Part model, mm, in its own coordinate system. A direction names the side the tool comes from. Coordinates: 2 decimals unless noted, no trailing zeros. Loops run counter-clockwise (first coordinate to the right, second up) from the corner with the lowest first, then second, coordinate; pieces in that order, holes last. Notation, with made-up numbers: (2, -37.5) -> (37, -37.5) arc R9 cw to (37, -27.5) -> close; hole circle Ø1 at (24, 54). An arc over 180 degrees is marked (long way). Use one line per item in the form item = value. Start each with the question number.
(1) Band-saw the part on C-C on y = 26. Give the cut face in (x, z).
(2) 3-axis set-ups, long thin cutter, end or side, ignore diameter. For faces 5 (the flat face through (42.92, 19.18, -0.03)), 6 (the flat face through (43, 32, 0)): which of +Z, -Z, +X, -X, +Y, -Y reach the whole face in a straight line?
(3) Band-saw the part on D-D on x = 14. Give the cut face in (y, z), then the cut area to 3 significant figures.
(4) Mould opens along X. For faces 1 (the cylindrical face through (48.7, 21.833, -0.028)), 2 (the flat face through (24, 18, 2)), 3 (the cylindrical face through (18.821, 14.546, 0.028)), 4 (the flat face through (52.17, 24.97, -0.03)) say: +X half, -X half, draft (parallel to the pull), parting line (faces both ways), or undercut.
(5) Pin check, flat tip, straight feed: P1, Ø3, axis at x = 0, y = 0, coming from the +Z side. Stop position of the tip, or through.
(6) Drill centre lines: L1, parallel to X at y = 27, z = -1.45; L2, parallel to Y at x = 3, z = 0.3; L3, parallel to X at y = 20, z = -0.65. Where is each one in solid material? Low to high. Write a range as [from, to].
(7) Band-saw the part on B-B on x = 0. Give the cut face in (y, z).
(8) Band-saw the part on A-A on z = -1.1. Give the cut face in (x, y), then the cut area to 3 significant figures.
```python
from build123d import *

# Parameters (mm, degrees)
BOSS_EXTRUDE1_DEPTH      = 2
BOSS_EXTRUDE1_DEPTH_BACK = 2
SKETCH2_R                = 1.55
FILLET1_R                = 20
BOSS_EXTRUDE3_START      = -4
BOSS_EXTRUDE3_DEPTH      = 4
FILLET3_R                = 6


with BuildPart() as part:
    # Sketch2 → Boss-Extrude1 (new, two sides: drawn at the far end of the back side and taken through both)
    with BuildSketch(Plane.XY.offset(-BOSS_EXTRUDE1_DEPTH_BACK)):
        with BuildLine():
            Line((1.575752274, -4.745208612), (38.598254294, 14.069940073))
            Line((38.598254294, 14.069940073), (44.683748534, 21.26396825))
            ThreePointArc((44.683748534, 21.26396825), (46.605489471, 28.139740122), (40.590896347, 31.986036602))
            Line((40.590896347, 31.986036602), (3, 31))
            ThreePointArc((3, 31), (-1.722747684, 24.35815521), (6.101607472, 22.078261726))
            Line((6.101607472, 22.078261726), (26.170960727, 22.604695486))
            Line((26.170960727, 22.604695486), (19.115779569, 14.264342174))
            Line((19.115779569, 14.264342174), (0.76923556, 4.940473323))
            ThreePointArc((0.76923556, 4.940473323), (-4.982755324, -0.41490888), (1.575752274, -4.745208612))
        make_face()
        Circle(SKETCH2_R, mode=Mode.SUBTRACT)
        with Locations((41, 26)):
            Circle(SKETCH2_R, mode=Mode.SUBTRACT)
        with Locations((3, 26)):
            Circle(SKETCH2_R, mode=Mode.SUBTRACT)
    extrude(amount=BOSS_EXTRUDE1_DEPTH + BOSS_EXTRUDE1_DEPTH_BACK)

    # Fillet1
    fillet1_edges = [part.edges().sort_by_distance(p)[0] for p in [
        (38.598254294, 14.069940073, 0),
        (19.115779569, 14.264342174, 0),
    ]]
    fillet(fillet1_edges, radius=FILLET1_R)

    # Sketch4 → Boss-Extrude3 (add)
    with BuildSketch(Plane.XY.offset(2).offset(BOSS_EXTRUDE3_START)):
        with BuildLine():
            Line((44.683748534, 21.26396825), (47.128315366, 17.33721301))
            ThreePointArc((47.128315366, 17.33721301), (49.590140611, 15.561753741), (52.589716544, 16.025847893))
            Line((52.589716544, 16.025847893), (52.014355474, 16.847548658))
            ThreePointArc((52.014355474, 16.847548658), (48.803326553, 21.908657431), (52.460976548, 17.160276102))
            Line((52.460976548, 17.160276102), (53.036337618, 16.338575336))
            ThreePointArc((53.036337618, 16.338575336), (54.438800344, 18.629754015), (54.07561509, 21.291426028))
            Line((54.07561509, 21.291426028), (48.52701486, 31.999999837))
            Line((48.52701486, 31.999999837), (41.001398133, 31.999999837))
            ThreePointArc((41.001398133, 31.999999837), (46.67544448, 27.946620135), (44.683748534, 21.26396825))
        make_face()
    extrude(amount=BOSS_EXTRUDE3_DEPTH)

    # Fillet3
    fillet3_edges = [part.edges().sort_by_distance(p)[0] for p in [
        (48.52701486, 31.999999837, 0),
    ]]
    fillet(fillet3_edges, radius=FILLET3_R)


solid = part.part
```
A:
q1.outline = (-2, -2) -> (1.45, -2) -> (1.45, 2) -> (-2, 2) -> close; (4.55, -2) -> (39.45, -2) -> (39.45, 2) -> (4.55, 2) -> close; (42.55, -2) -> (51.64, -2) -> (51.64, 2) -> (42.55, 2) -> close
q2.face_5 = +Z, -Z, -Y
q2.face_6 = +Z, -Z, +X, -X, +Y
q3.outline = (1.57, -2) -> (11.66, -2) -> (11.66, 2) -> (1.57, 2) -> close; (22.29, -2) -> (31.29, -2) -> (31.29, 2) -> (22.29, 2) -> close
q3.area = 76.4 mm²
q4.face_1 = undercut
q4.face_2 = draft
q4.face_3 = -X half
q4.face_4 = +X half
q5.P1 = through
q6.L1 = [-1.9, 1.82], [4.18, 39.82], [42.18, 51.12]
q6.L2 = [-4.02, 6.07], [21, 24.45], [27.55, 31]
q6.L3 = [23.97, 43.61], [45.47, 47.57], [53.47, 54.49]
q7.outline = (-5, -2) -> (-1.55, -2) -> (-1.55, 2) -> (-5, 2) -> close; (1.55, -2) -> (5, -2) -> (5, 2) -> (1.55, 2) -> close; (22, -2) -> (30, -2) -> (30, 2) -> (22, 2) -> close
q8.outline = (0.77, 4.94) arc R5 ccw (long way) to (1.58, -4.75) -> (35, 12.24) arc R20 ccw to (41.21, 17.15) -> (44.68, 21.26) -> (47.13, 17.34) arc R4 ccw to (52.59, 16.03) -> (52.01, 16.85) arc R3 cw (long way) to (52.46, 17.16) -> (53.04, 16.34) arc R4 ccw to (54.08, 21.29) -> (50.21, 28.76) arc R6 ccw to (44.88, 32) -> (41, 32) arc R6 ccw to (40.59, 31.99) -> (3, 31) arc R5 ccw (long way) to (6.1, 22.08) -> (26.17, 22.6) -> (21.72, 17.35) arc R20 cw to (15.52, 12.43) -> close; hole circle Ø3.1 at (0, 0); hole circle Ø3.1 at (3, 26); hole circle Ø3.1 at (41, 26)
q8.area = 976 mm²
